from build123d import *

# Parameters (mm, degrees)
SKETCH1_W                 = 16.6158
SKETCH1_H                 = 27.2711
SKETCH1_W_2               = 12.6158
SKETCH1_H_2               = 23.2711
BOSS_EXTRUDE1_DEPTH       = 8
SKETCH2_W                 = 3.8956
SKETCH2_H                 = 2.5
CUT_EXTRUDE2_DEPTH        = 27.165323553
SKETCH5_W                 = 16
SKETCH5_H                 = 23.53
BOSS_EXTRUDE2_DEPTH       = 0.0001
M2_CLEARANCE_HOLE1_REACH  = 28.452
M2_CLEARANCE_HOLE1_BORE_R = 1.2
BOSS_EXTRUDE3_DEPTH       = 3.5
SKETCH9_W                 = 16
SKETCH9_H                 = 23.53
BOSS_EXTRUDE4_DEPTH       = 1.5
SKETCH10_R                = 2.35
CUT_EXTRUDE3_DEPTH        = 1.5
FILLET1_R                 = 1
BOSS_EXTRUDE5_DEPTH       = 16


with BuildPart() as part:
    # Sketch1 → Boss-Extrude1 (new, symmetric)
    with BuildSketch(Plane(origin=(0, 0, 0), x_dir=(0, 0, -1), z_dir=(1, 0, 0))):
        with Locations((0, -5.32765)):
            Rectangle(SKETCH1_W, SKETCH1_H)
        with Locations((0, -5.32765)):
            Rectangle(SKETCH1_W_2, SKETCH1_H_2, mode=Mode.SUBTRACT)
    extrude(amount=BOSS_EXTRUDE1_DEPTH, both=True)

    # Sketch2 → Cut-Extrude2 (cut, through all)
    with BuildSketch(Plane.ZY.offset(8)):
        with Locations((0, 6.8079)):
            Rectangle(SKETCH2_W, SKETCH2_H)
    extrude(amount=-CUT_EXTRUDE2_DEPTH, mode=Mode.SUBTRACT)

    # Sketch5 → Boss-Extrude2 (add)
    with BuildSketch(Plane.XY.offset(8.3079)):
        with Locations((0, -7.1982)):
            Rectangle(SKETCH5_W, SKETCH5_H)
    extrude(amount=BOSS_EXTRUDE2_DEPTH)

    # M2 Clearance Hole1 bore → M2 Clearance Hole1 (cut, up to next)
    with BuildSketch(Plane.XY.offset(8.308), mode=Mode.PRIVATE) as m2_clearance_hole1_sk1:
        with Locations((3.28, 0.4168)):
            Circle(M2_CLEARANCE_HOLE1_BORE_R)
    m2_clearance_hole1_tool1 = extrude(m2_clearance_hole1_sk1.sketch, amount=-M2_CLEARANCE_HOLE1_REACH, mode=Mode.PRIVATE) & part.part
    # M2 Clearance Hole1 bore → M2 Clearance Hole1 (cut, up to next)
    with BuildSketch(Plane.XY.offset(8.308), mode=Mode.PRIVATE) as m2_clearance_hole1_sk2:
        with Locations((3.28, -14.8132)):
            Circle(M2_CLEARANCE_HOLE1_BORE_R)
    m2_clearance_hole1_tool2 = extrude(m2_clearance_hole1_sk2.sketch, amount=-M2_CLEARANCE_HOLE1_REACH, mode=Mode.PRIVATE) & part.part
    add(m2_clearance_hole1_tool1.solids().sort_by_distance((3.28, 0.4168, 8.308))[0], mode=Mode.SUBTRACT)
    add(m2_clearance_hole1_tool2.solids().sort_by_distance((3.28, -14.8132, 8.308))[0], mode=Mode.SUBTRACT)

    # Sketch8 → Boss-Extrude3 (add)
    with BuildSketch(Plane.XY.offset(8.308)):
        with BuildLine():
            Line((-8, -17.8132), (3.11, -17.8132))
            ThreePointArc((3.11, -17.8132), (5.245462479, -16.928662479), (6.13, -14.7932))
            Line((6.13, -14.7932), (6.13, 0.3968))
            ThreePointArc((6.13, 0.3968), (5.245462479, 2.532262479), (3.11, 3.4168))
            Line((3.11, 3.4168), (-8, 3.4168))
            Line((-8, 3.4168), (-8, 4.5668))
            Line((-8, 4.5668), (8, 4.5668))
            Line((8, 4.5668), (8, -18.9632))
            Line((8, -18.9632), (-8, -18.9632))
            Line((-8, -18.9632), (-8, -17.8132))
        make_face()
    extrude(amount=BOSS_EXTRUDE3_DEPTH)

    # Sketch9 → Boss-Extrude4 (add)
    with BuildSketch(Plane.XY.offset(11.808)):
        with Locations((0, -7.1982)):
            Rectangle(SKETCH9_W, SKETCH9_H)
    extrude(amount=BOSS_EXTRUDE4_DEPTH)

    # Sketch10 → Cut-Extrude3 (cut)
    with BuildSketch(Plane.XY.offset(13.308)):
        with Locations((3.28, 0.4168)):
            Circle(SKETCH10_R)
        with Locations((3.28, -14.8132)):
            Circle(SKETCH10_R)
        with BuildLine():
            Line((-3.335, -5.1982), (-0.335, -5.1982))
            ThreePointArc((-0.335, -5.1982), (1.665, -7.1982), (-0.335, -9.1982))
            Line((-0.335, -9.1982), (-3.335, -9.1982))
            ThreePointArc((-3.335, -9.1982), (-5.335, -7.1982), (-3.335, -5.1982))
        make_face()
    extrude(amount=-CUT_EXTRUDE3_DEPTH, mode=Mode.SUBTRACT)

    # Fillet1
    fillet1_edges = [part.edges().sort_by_distance(p)[0] for p in [
        (8, -7.1982, 13.308),
        (0, 4.5668, 13.308),
        (0, -18.9632, 13.308),
        (8, -18.9632, 2.50005),
        (0, 8.3079, 8.3079),
        (8, 4.5668, 10.80795),
    ]]
    fillet(fillet1_edges, radius=FILLET1_R)

    # Sketch11 → Boss-Extrude5 (add)
    with BuildSketch(Plane.ZY.offset(8)):
        Polygon((2.9478, 8.3079), (1.9478, 9.3079), (-1.9478, 9.3079), (-2.9478, 8.3079), align=None)
    extrude(amount=-BOSS_EXTRUDE5_DEPTH)


solid = part.part
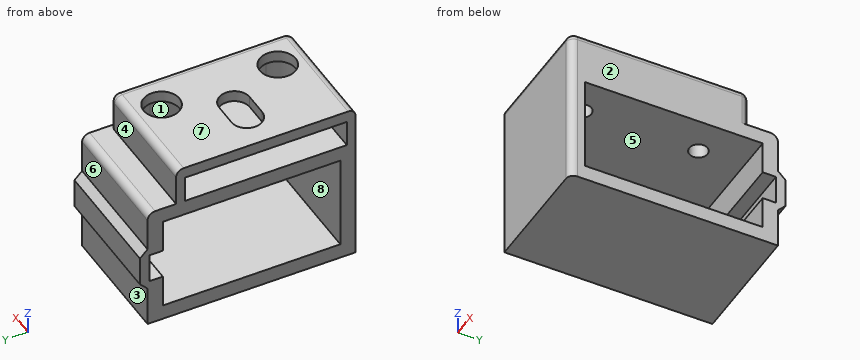
Input: part model. Units: mm. Frame: model coordinates. Face numbers are marked on the shaded views. A direction names the side the tool comes from. Coordinates: 2 decimals unless noted, no trailing zeros. Loops run counter-clockwise (first coordinate to the right, second up) from the corner with the lowest first, then second, coordinate; pieces in that order, holes last. Notation, with made-up numbers: (27.25, -7.5) - (72.25, -7.5) arc R14 ccw to (72.25, 17.5) - close; hole circle Ø7 at (20, 67). An arc over 180 degrees is marked (long way). Answer in a Markdown table with one row per item. Add a question column.
Item 1: Mould query, pull axis Z, two halves, no side actions, for the marked faces 6, 7 and 8. Classes: released by +Z, released by -Z, zero draft, split by the parting line, or undercut.
Item 2: Access query for the marked faces 1, 2, 3, 4 and 5. Directions: +Z, -Z, +X, -X, +Y, -Y. A direction counts if a zero-diameter tool reaches every point of the face in a straight line with its end or side. Return the directions, or none.
Item 3: Section query A-A on z = 0.25. Return the cut outline in (x, y), then the cut area to 3 significant figures.
Item 4: Contact query for flat-ended pins moving along their axis: P1, Ø2.5, axis at x = -2, z = -6.5, coming from the +Y side; P2, Ø10, axis at y = -4, z = 4, coming from the -X side; P3, Ø0.9, axis at x = 0, y = 7, coming from the +Z side; P4, Ø1.6, axis at x = -2.5, z = 12.5, coming from the +Y side. Output: stop coordinate, or through.
Item 5: Section query C-C on y = -16.5. Return the cut outline in (x, z).
Item 6: Line query: line 1 along Z through (x, y) = (-7, -14.5); line 2 along Y through (x, z) = (2.25, 1); line 3 along Z through (x, y) = (-4.5, 7). Output: solid intervals per line, ascending. Write a range as [from, to].
Item 7: Section query D-D on z = 4.5. Return the cut outline in (x, y).
Recorded:
| question | item | result |
|---|---|---|
| 1 | face 6 | zero draft |
| 1 | face 7 | released by +Z |
| 1 | face 8 | undercut |
| 2 | face 1 | -X |
| 2 | face 2 | +Z, -Z, +X, +Y, -Y |
| 2 | face 3 | -Z, +X, -X, +Y |
| 2 | face 4 | +Z, +X, -X, +Y |
| 2 | face 5 | +X, -X |
| 3 | outline | (-8, -18.96) - (7, -18.96) arc R1 ccw to (8, -17.96) - (8, -16.96) - (-8, -16.96) - close; (-8, 8.06) - (8, 8.06) - (8, 9.31) - (-8, 9.31) - close |
| 3 | area | 51.8 mm^2 |
| 4 | P1 | y = 8.31 |
| 4 | P2 | x = -8 |
| 4 | P3 | z = 8.31 |
| 4 | P4 | y = 4.57 |
| 5 | outline | (-8, -8.31) - (8, -8.31) - (8, -6.31) - (-8, -6.31) - close; (-8, 6.31) - (8, 6.31) - (8, 12.31) arc R1 ccw to (7, 13.31) - (4.92, 13.31) - (4.92, 11.81) - (5.6, 11.81) - (5.6, 8.31) - (-8, 8.31) - close; (-8, 11.81) - (1.64, 11.81) - (1.64, 13.31) - (-8, 13.31) - close |
| 6 | line 1 | [-8.31, -6.31], [6.31, 8.31], [11.81, 13.31] |
| 6 | line 2 | [-18.96, -16.96], [8.06, 9.31] |
| 6 | line 3 | [-8.31, -1.95], [1.95, 8.31] |
| 7 | outline | (-8, -18.96) - (7, -18.96) arc R1 ccw to (8, -17.96) - (8, -16.96) - (-8, -16.96) - close; (-8, 6.31) - (8, 6.31) - (8, 8.31) - (-8, 8.31) - close |
